Build history of the part. All positions in model axes, mm. Face numbers are marked on the shaded views. A direction names the side the tool comes from. Give positions to 0.01 mm unless a question says otherwise; leave off trailing zeros. Loops run counter-clockwise (first coordinate to the right, second up) from the corner with the lowest first, then second, coordinate; pieces in that order, holes last. Notation, with made-up numbers: (3, 65) -> (7, 65) arc R23 cw to (7, 82) -> close; hole circle Ø7 at (-26.5, 12.25). An arc over 180 degrees is marked (long way). Answer as a JSON object with one key per item and string values. Group by question number.
Q1. Band-saw the part on D-D, the plane y = -2.5. Write the cut outline in (x, z).
Q2. Tool access for the marked faces 1 and 2: list every direction of +Z, -Z, +X, -X, +Y, -Y with a clear straight run to the whole face (end or side of a thin tool).
Q3. Wall check: probe 1 along Z at (x, y) = (-13.5, 8.65); probe 2 along X at (y, z) = (-3.25, 7); probe 3 along Y at (x, z) = (-1.25, 7.5). Give the ranges that are in metal, low to high. Write a range as from..to.
Q4. Band-saw the part on B-B, the plane y = -5. Write the cut outline in (x, z), plus the area to 3 significant figures.
Q5. Drop flat-ended pins along their axis: pin 1 (1 mm diameter, centred on y = 6, z = 3.5, fed in from -X); pin 2 (1 mm diameter, centred on x = -6, z = 4, fed in from -Y). Give the stop position or say it passes through.
Q6. Band-saw the part on C-C, the plane x = -13.5. Write the cut outline in (y, z).
Q7. Band-saw the part on A-A, the plane z = 4. Write the cut outline in (x, y).
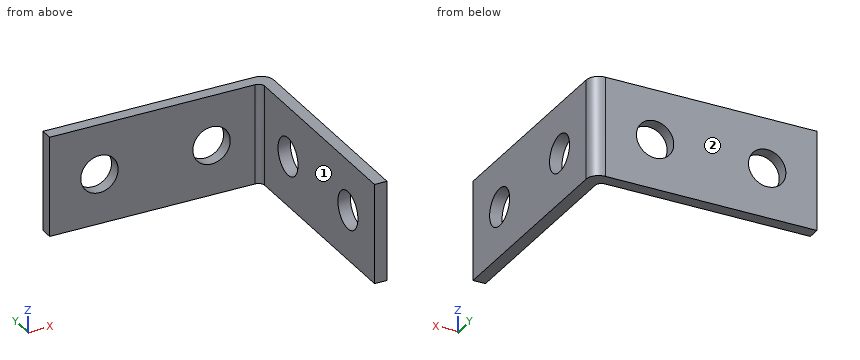
from build123d import *

# Parameters (mm, degrees)
F0_W     = 1
F0_H     = 1
F0_W_2   = 17
F0_H_2   = 17
F1_DEPTH = 8
F3_R     = 1.5
F4_DEPTH = 25
F2_R     = 1.5
F5_DEPTH = 25
F6_R     = 1
F7_R     = 0.5


with BuildPart() as f1:
    # F0 (on Top) → F1 (new body)
    with BuildSketch(Plane.XY):
        with Locations((0, 8.5)):
            Rectangle(F0_W, F0_H)
        with Locations((-9, 8.5)):
            Rectangle(F0_W_2, F0_H)
        with Locations((0, -0.5)):
            Rectangle(F0_W, F0_H_2)
    extrude(amount=F1_DEPTH)

    # F3 (on face) → F4 (cut)
    with BuildSketch(Plane.XZ.offset(-8)):
        with BuildLine():
            ThreePointArc((-15, 4), (-13.5, 2.5), (-12, 4))
            ThreePointArc((-12, 4), (-13.5, 5.5), (-15, 4))
        make_face()
        with Locations((-4.5, 4)):
            Circle(F3_R)
    extrude(amount=-F4_DEPTH, mode=Mode.SUBTRACT)

    # F2 (on face) → F5 (cut)
    with BuildSketch(Plane(origin=(-0.5, 0, 0), x_dir=(0, -1, 0), z_dir=(-1, 0, 0))):
        with Locations((5, 4)):
            Circle(F2_R)
        with Locations((-4, 4)):
            Circle(F2_R)
    extrude(amount=-F5_DEPTH, mode=Mode.SUBTRACT)

    # F6
    f6_edges = [f1.edges().sort_by_distance(p)[0] for p in [
        (0.5, 9, 4),
    ]]
    fillet(f6_edges, radius=F6_R)

    # F7
    f7_edges = [f1.edges().sort_by_distance(p)[0] for p in [
        (-0.5, 8, 4),
    ]]
    fillet(f7_edges, radius=F7_R)


solid = f1.part
Worked answers:
{
 "1": {"outline": "(-0.5, 0) -> (0.5, 0) -> (0.5, 8) -> (-0.5, 8) -> close"},
 "2": {"face 1": "+Z, -Z, -X, -Y", "face 2": "+Z, -Z, +X, -X, +Y"},
 "3": {"probe 1": "0..2.5, 5.5..8", "probe 2": "-0.5..0.5", "probe 3": "8..9"},
 "4": {"outline": "(-0.5, 0) -> (0.5, 0) -> (0.5, 2.5) -> (-0.5, 2.5) -> close; (-0.5, 5.5) -> (0.5, 5.5) -> (0.5, 8) -> (-0.5, 8) -> close", "area": "5.00 mm2"},
 "5": {"pin 1": "x = -0.5", "pin 2": "y = 8"},
 "6": {"outline": "(8, 0) -> (9, 0) -> (9, 2.5) -> (8, 2.5) -> close; (8, 5.5) -> (9, 5.5) -> (9, 8) -> (8, 8) -> close"},
 "7": {"outline": "(-17.5, 8) -> (-15, 8) -> (-15, 9) -> (-17.5, 9) -> close; (-12, 8) -> (-6, 8) -> (-6, 9) -> (-12, 9) -> close; (-3, 8) -> (-1, 8) arc R0.5 cw to (-0.5, 7.5) -> (-0.5, 5.5) -> (0.5, 5.5) -> (0.5, 8) arc R1 ccw to (-0.5, 9) -> (-3, 9) -> close; (-0.5, -9) -> (0.5, -9) -> (0.5, -6.5) -> (-0.5, -6.5) -> close; (-0.5, -3.5) -> (0.5, -3.5) -> (0.5, 2.5) -> (-0.5, 2.5) -> close"}
}
